```python
from build123d import *

# Parameters (mm, degrees)
SKETCH1_W           = 10
SKETCH1_H           = 16
BOSS_EXTRUDE1_DEPTH = 3
SKETCH2_W           = 10
SKETCH2_H           = 3
BOSS_EXTRUDE2_DEPTH = 5
SKETCH3_W           = 10
SKETCH3_H           = 7
BOSS_EXTRUDE3_DEPTH = 2
FILLET1_R           = 5
FILLET2_R           = 5
FILLET3_R           = 2
SKETCH4_R           = 1
CUT_EXTRUDE1_DEPTH  = 19.309833585


with BuildPart() as part:
    # Sketch1 → Boss-Extrude1 (new body)
    with BuildSketch(Plane.XZ.offset(-25)):
        with Locations((0, 2.5)):
            Rectangle(SKETCH1_W, SKETCH1_H)
    extrude(amount=BOSS_EXTRUDE1_DEPTH)

    # Sketch2 → Boss-Extrude2 (add)
    with BuildSketch(Plane.XZ.offset(-22)):
        with Locations((0, -4)):
            Rectangle(SKETCH2_W, SKETCH2_H)
        with Locations((0, 9)):
            Rectangle(SKETCH2_W, SKETCH2_H)
    extrude(amount=BOSS_EXTRUDE2_DEPTH)

    # Sketch3 → Boss-Extrude3 (add)
    with BuildSketch(Plane.XZ.offset(-17)):
        with Locations((0, 11)):
            Rectangle(SKETCH3_W, SKETCH3_H)
        with Locations((0, -6)):
            Rectangle(SKETCH3_W, SKETCH3_H)
    extrude(amount=BOSS_EXTRUDE3_DEPTH)

    # Fillet1
    fillet1_edges = [part.edges().sort_by_distance(p)[0] for p in [
        (0, 22, 7.5),
        (0, 22, -2.5),
    ]]
    fillet(fillet1_edges, radius=FILLET1_R - 0.0001)  # a hair under: the kernel refuses the full size

    # Fillet2
    fillet2_edges = [part.edges().sort_by_distance(p)[0] for p in [
        (0, 15, -2.5),
        (0, 15, 7.5),
    ]]
    fillet(fillet2_edges, radius=FILLET2_R)

    # Fillet3
    fillet3_edges = [part.edges().sort_by_distance(p)[0] for p in [
        (0, 17, -5.5),
        (0, 17, 10.5),
    ]]
    fillet(fillet3_edges, radius=FILLET3_R)

    # Sketch4 → Cut-Extrude1 (cut, through all)
    with BuildSketch(Plane(origin=(0, 25, 0), x_dir=(1, 0, 0), z_dir=(0, 1, 0))):
        with Locations(Location((0, 1.5, 0), (0, 0, 270))):
            Circle(SKETCH4_R)
        with Locations(Location((0, -6.5, 0), (0, 0, 270))):
            Circle(SKETCH4_R)
    extrude(amount=-CUT_EXTRUDE1_DEPTH, mode=Mode.SUBTRACT)


solid = part.part
```
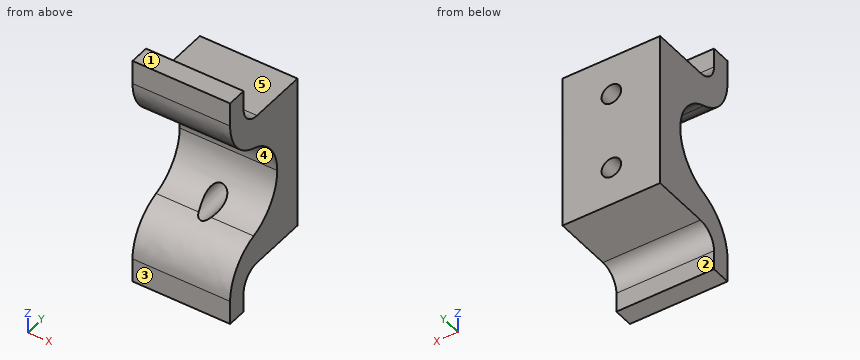
Can you work these out from the model? Positions are in its coordinate system, mm. Face numbers are marked on the shaded views. A direction names the side the tool comes from. Coordinates: 2 decimals unless noted, no trailing zeros. Loops run counter-clockwise (first coordinate to the right, second up) from the corner with the lowest first, then second, coordinate; pieces in that order, holes last.
Item 1: I'm going to push flat-ended pins straight in: pin 1 (2.5 mm diameter, centred on x = 0, z = -1.5, fed in from -Y); pin 2 (3 mm diameter, centred on x = -2, y = 23, fed in from -Z); pin 3 (2 mm diameter, centred on x = 1, z = 14, fed in from +Y). Where does each tip first touch, or does it pass through?
Answers below:
pin 1: stops at y = 17.43
pin 2: stops at z = -5.5
pin 3: stops at y = 17
Item 2: Please list where these lines run through material, in increasing order: L1, parallel to Z at x = 0, y = 22.75; L2, parallel to Z at x = 0, y = 21.25; L3, parallel to X at y = 23.75, z = -1.5.
Answers below:
L1: z = -5.5 to -2.5, -0.5 to 5.5, 7.5 to 10.5
L2: z = -5.5 to -2.5, -0.5 to -0.13, 5.13 to 5.5, 7.5 to 10.5
L3: x = -5 to -1, 1 to 5
Item 3: Suppose I cut it at D-D (x = 0). State how many separate pieces and enclosed holes the cut face has, then the cut area to 3 significant figures.
Answers below:
separate pieces: 3
enclosed holes: 0
area: 90.2 mm2
Item 4: Suppose I cut it at C-C (z = -7.75). Please give me the cut outline in (x, y), then the cut area to 3 significant figures.
Answers below:
outline: (-5, 15) - (5, 15) - (5, 17) - (-5, 17) - close
area: 20.0 mm2
Item 5: Suppose I cut it at B-B (z = 6.5). Please give me the cut outline in (x, y).
Answers below:
outline: (-5, 20) - (-1, 20) - (-1, 25) - (-5, 25) - close; (1, 20) - (5, 20) - (5, 25) - (1, 25) - close
Item 6: Suppose I cut it at A-A (y = 21.5). Please give me the cut outline in (x, z).
Answers below:
outline: (-5, -5.5) - (5, -5.5) - (5, 0.32) - (-5, 0.32) - close; (-5, 4.68) - (5, 4.68) - (5, 10.5) - (-5, 10.5) - close; hole circle Ø2 at (0, -1.5); hole circle Ø2 at (0, 6.5)
Item 7: Which directions (+Z, -Z, +X, -X, +Y, -Y) give clear straight access to the entire face, cutting with the end or side of a thin tool? Please do the marked faces 1, 2, 3, 4 and 5.
Answers below:
face 1: +Z, +X, -X, +Y, -Y
face 2: -Z, +X, -X, +Y
face 3: +Z, -Z, +X, -X, -Y
face 4: +X, -X, -Y
face 5: +Z, +X, -X, +Y
